```python
from build123d import *

# Parameters (mm, degrees)
BOSS_EXTRUDE1_DEPTH = 1
BOSS_EXTRUDE2_DEPTH = 2.7
SKETCH5_OUTSIDE_W   = 198.872
SKETCH5_OUTSIDE_H   = 130.378
SKETCH5_OUTSIDE_R   = 3
CUT_EXTRUDE1_DEPTH  = 2
BOSS_EXTRUDE3_DEPTH = 0.5
BOSS_EXTRUDE4_DEPTH = 1
CUT_EXTRUDE2_START  = 0.5
SKETCH9_R           = 14.807450978
CUT_EXTRUDE2_DEPTH  = 0.5


with BuildPart() as part:
    # Sketch3 → Boss-Extrude1 (new body)
    with BuildSketch(Plane(origin=(0, 0, 0), x_dir=(1, 0, 0), z_dir=(0, 1, 0))):
        Polygon((-80, 45), (80, 45), (80, -46.505636843), (-80, -45), align=None)
    extrude(amount=BOSS_EXTRUDE1_DEPTH)

    # Sketch4 → Boss-Extrude2 (add)
    with BuildSketch(Plane.XZ):
        with BuildLine():
            Line((-70.35, 37.979513383), (-70.35, 32.020486617))
            add(Edge.make_bspline(
                [(-70.35, 37.979513383), (-73.35, 37.979513383), (-73.35, 35), (-73.35, 32.020486617), (-70.35, 32.020486617)],
                knots=[4.71238898, 4.71238898, 4.71238898, 6.283185307, 6.283185307, 7.853981634, 7.853981634, 7.853981634], degree=2, weights=[1, 0.707106781, 1, 0.707106781, 1]))
        make_face()
        with BuildLine():
            Line((-69.65, 37.979513383), (-69.65, 32.020486617))
            add(Edge.make_bspline(
                [(-69.65, 32.020486617), (-66.65, 32.020486617), (-66.65, 35), (-66.65, 37.979513383), (-69.65, 37.979513383)],
                knots=[4.71238898, 4.71238898, 4.71238898, 6.283185307, 6.283185307, 7.853981634, 7.853981634, 7.853981634], degree=2, weights=[1, 0.707106781, 1, 0.707106781, 1]))
        make_face()
        with BuildLine():
            Line((69.65, 37.979513383), (69.65, 32.020486617))
            add(Edge.make_bspline(
                [(69.65, 37.979513383), (66.65, 37.979513383), (66.65, 35), (66.65, 32.020486617), (69.65, 32.020486617)],
                knots=[4.71238898, 4.71238898, 4.71238898, 6.283185307, 6.283185307, 7.853981634, 7.853981634, 7.853981634], degree=2, weights=[1, 0.707106781, 1, 0.707106781, 1]))
        make_face()
        with BuildLine():
            Line((70.35, 37.979513383), (70.35, 32.020486617))
            add(Edge.make_bspline(
                [(70.35, 32.020486617), (73.35, 32.020486617), (73.35, 35), (73.35, 37.979513383), (70.35, 37.979513383)],
                knots=[4.71238898, 4.71238898, 4.71238898, 6.283185307, 6.283185307, 7.853981634, 7.853981634, 7.853981634], degree=2, weights=[1, 0.707106781, 1, 0.707106781, 1]))
        make_face()
        with BuildLine():
            Line((69.65, -32.020486617), (69.65, -37.979513383))
            add(Edge.make_bspline(
                [(69.65, -32.020486617), (66.65, -32.020486617), (66.65, -35), (66.65, -37.979513383), (69.65, -37.979513383)],
                knots=[4.71238898, 4.71238898, 4.71238898, 6.283185307, 6.283185307, 7.853981634, 7.853981634, 7.853981634], degree=2, weights=[1, 0.707106781, 1, 0.707106781, 1]))
        make_face()
        with BuildLine():
            Line((70.35, -32.020486617), (70.35, -37.979513383))
            add(Edge.make_bspline(
                [(70.35, -37.979513383), (73.35, -37.979513383), (73.35, -35), (73.35, -32.020486617), (70.35, -32.020486617)],
                knots=[4.71238898, 4.71238898, 4.71238898, 6.283185307, 6.283185307, 7.853981634, 7.853981634, 7.853981634], degree=2, weights=[1, 0.707106781, 1, 0.707106781, 1]))
        make_face()
        with BuildLine():
            Line((-70.35, -32.020486617), (-70.35, -37.979513383))
            add(Edge.make_bspline(
                [(-70.35, -32.020486617), (-73.35, -32.020486617), (-73.35, -35), (-73.35, -37.979513383), (-70.35, -37.979513383)],
                knots=[4.71238898, 4.71238898, 4.71238898, 6.283185307, 6.283185307, 7.853981634, 7.853981634, 7.853981634], degree=2, weights=[1, 0.707106781, 1, 0.707106781, 1]))
        make_face()
        with BuildLine():
            Line((-69.65, -32.020486617), (-69.65, -37.979513383))
            add(Edge.make_bspline(
                [(-69.65, -37.979513383), (-66.65, -37.979513383), (-66.65, -35), (-66.65, -32.020486617), (-69.65, -32.020486617)],
                knots=[4.71238898, 4.71238898, 4.71238898, 6.283185307, 6.283185307, 7.853981634, 7.853981634, 7.853981634], degree=2, weights=[1, 0.707106781, 1, 0.707106781, 1]))
        make_face()
    extrude(amount=BOSS_EXTRUDE2_DEPTH)

    # Sketch5 outside → Cut-Extrude1 (cut)
    with BuildSketch(Plane.XZ):
        with Locations((0, 0.753)):
            Rectangle(SKETCH5_OUTSIDE_W, SKETCH5_OUTSIDE_H)
        with Locations((-70, 35)):
            Circle(SKETCH5_OUTSIDE_R, mode=Mode.SUBTRACT)
        with Locations((70, 35)):
            Circle(SKETCH5_OUTSIDE_R, mode=Mode.SUBTRACT)
        with Locations((70, -35)):
            Circle(SKETCH5_OUTSIDE_R, mode=Mode.SUBTRACT)
        with Locations((-70, -35)):
            Circle(SKETCH5_OUTSIDE_R, mode=Mode.SUBTRACT)
    extrude(amount=CUT_EXTRUDE1_DEPTH, mode=Mode.SUBTRACT)

    # Sketch7 → Boss-Extrude3 (add)
    with BuildSketch(Plane(origin=(0, 1, 0), x_dir=(1, 0, 0), z_dir=(0, 1, 0))):
        with BuildLine():
            Line((-54.317045104, 39.602220595), (2.604668629, 39.602220595))
            ThreePointArc((2.604668629, 39.602220595), (16.151568109, -36.252545046), (-31.185365289, 24.547773147))
            Line((-31.185365289, 24.547773147), (-45.57985147, 24.320826837))
            Line((-45.57985147, 24.320826837), (-54.317045104, 39.602220595))
        make_face()
    extrude(amount=BOSS_EXTRUDE3_DEPTH)

    # Sketch8 → Boss-Extrude4 (add)
    with BuildSketch(Plane(origin=(0, 1, 0), x_dir=(1, 0, 0), z_dir=(0, 1, 0))):
        with BuildLine():
            Line((-39.773980052, 25.288720826), (-33.810282359, 14.830937097))
            Line((-33.810282359, 14.830937097), (-20.815447328, 14.373801562))
            ThreePointArc((-20.815447328, 14.373801562), (12.021833569, -22.256786301), (-0.607961992, 25.288720826))
            Line((-0.607961992, 25.288720826), (-39.773980052, 25.288720826))
        make_face()
    extrude(amount=BOSS_EXTRUDE4_DEPTH)

    # Sketch9 → Cut-Extrude2 (cut)
    with BuildSketch(Plane(origin=(0, 1, 0), x_dir=(1, 0, 0), z_dir=(0, 1, 0)).offset(CUT_EXTRUDE2_START)):
        with Locations(Location((0, 0, 0), (0, 0, 270))):
            Circle(SKETCH9_R)
    extrude(amount=CUT_EXTRUDE2_DEPTH, mode=Mode.SUBTRACT)


solid = part.part
```
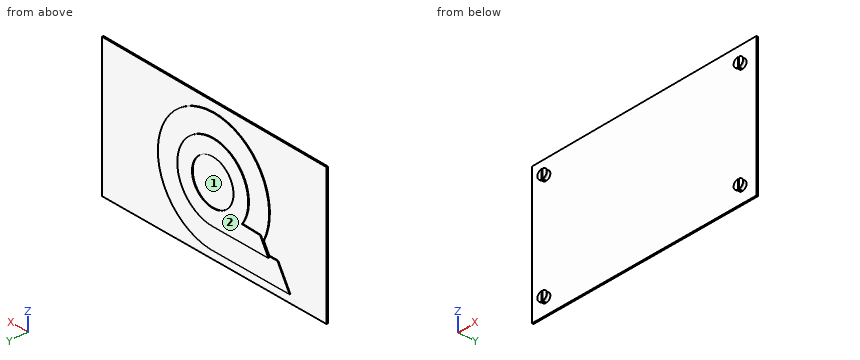
Can you work these out from the model? Positions are in its coordinate system, mm. Face numbers are marked on the shaded views. Coordinates: 2 decimals unless noted, no trailing zeros. Loops run counter-clockwise (first coordinate to the right, second up) from the corner with the lowest first, then second, coordinate; pieces in that order, holes last.
Item 1: Suppose I cut it at D-D (z = 30.5). Please give me the cut outline in (x, y), then the cut area to 3 significant figures.
Answers below:
outline: (-80, 0) - (80, 0) - (80, 1) - (25.39, 1) - (25.39, 1.5) - (-25.39, 1.5) - (-25.39, 1) - (-80, 1) - close
area: 185 mm2
Item 2: I'm going to push flat-ended pins straight in: pin 1 (3 mm diameter, centred on x = -36, z = 14, fed in from -Y); pin 2 (3.5 mm diameter, centred on x = -68, z = -34, fed in from +Y); pin 3 (10 mm diameter, centred on x = -4.5, z = -2, fed in from +Y). Where does each tip first touch, or does it pass through?
Answers below:
pin 1: stops at y = 0
pin 2: stops at y = 1
pin 3: stops at y = 1.5
Item 3: Suppose I cut it at B-B (z = 0). Please give me the cut outline in (x, y).
Answers below:
outline: (-80, 0) - (80, 0) - (80, 1) - (39.69, 1) - (39.69, 1.5) - (25.3, 1.5) - (25.3, 2) - (14.81, 2) - (14.81, 1.5) - (-14.81, 1.5) - (-14.81, 2) - (-25.3, 2) - (-25.3, 1.5) - (-39.69, 1.5) - (-39.69, 1) - (-80, 1) - close
Item 4: Suppose I cut it at C-C (x = -18.5). Please give me the cut outline in (y, z), then the cut area to 3 significant figures.
Answers below:
outline: (0, -45) - (1, -45) - (1, -39.6) - (1.5, -39.6) - (1.5, -25.29) - (2, -25.29) - (2, 17.25) - (1.5, 17.25) - (1.5, 35.11) - (1, 35.11) - (1, 45.58) - (0, 45.58) - close
area: 149 mm2
Item 5: Suppose I cut it at A-A (y = -0.8). Please give me the cut outline in (x, z).
Answers below:
outline: (-70.35, -37.98) - (-70.35, -32.02) arc R3 ccw to start; (-70.35, 32.02) - (-70.35, 37.98) arc R3 ccw to start; (-69.65, -37.98) arc R3 ccw to (-69.65, -32.02) - close; (-69.65, 32.02) arc R3 ccw to (-69.65, 37.98) - close; (69.65, -37.98) - (69.65, -32.02) arc R3 ccw to start; (69.65, 32.02) - (69.65, 37.98) arc R3 ccw to start; (70.35, -37.98) arc R3 ccw to (70.35, -32.02) - close; (70.35, 32.02) arc R3 ccw to (70.35, 37.98) - close
Item 6: Please list where these lines run through material, in increasing order: L1, parallel to X at y = -0.85, z = 34; L2, parallel to X at y = 1.8, z = 0; L3, parallel to Y at x = -50.5, z = -26.5.
Answers below:
L1: x = -72.83 to -70.35, -69.65 to -67.17, 67.17 to 69.65, 70.35 to 72.83
L2: x = -25.3 to -14.81, 14.81 to 25.3
L3: y = 0 to 1
Item 7: If we mould it in two halves opening along Z, with no side actions, what happens to the marked faces 1 and 2? For each: released by +Z, released by -Z, zero draft, split by the parting line, or undercut.
Answers below:
face 1: undercut
face 2: zero draft
